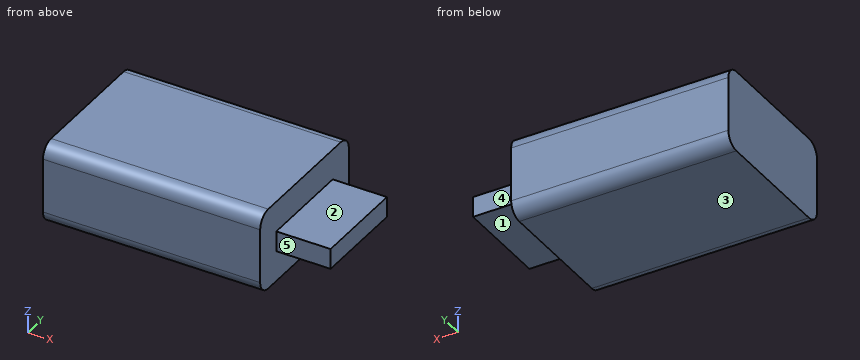
```python
from build123d import *

# Parameters (mm, degrees)
SKICA1_W                = 16
SKICA1_H                = 11
P_IDAT_VYSUNUT_M1_DEPTH = 6
ZAOBLIT1_R              = 1
SKICA2_W                = 1.5
SKICA2_H                = 7
P_IDAT_VYSUNUT_M2_DEPTH = 4


with BuildPart() as part:
    # Skica1 → Přidat vysunutím1 (new body)
    with BuildSketch(Plane.XY):
        Rectangle(SKICA1_W, SKICA1_H)
    extrude(amount=P_IDAT_VYSUNUT_M1_DEPTH)

    # Zaoblit1
    zaoblit1_edges = [part.edges().sort_by_distance(p)[0] for p in [
        (0, -5.5, 6),
        (0, -5.5, 0),
        (0, 5.5, 0),
        (0, 5.5, 6),
    ]]
    fillet(zaoblit1_edges, radius=ZAOBLIT1_R)

    # Skica2 → Přidat vysunutím2 (add)
    with BuildSketch(Plane(origin=(8, 0, 0), x_dir=(0, 0, -1), z_dir=(1, 0, 0))):
        with Locations((-3, 0)):
            Rectangle(SKICA2_W, SKICA2_H)
    extrude(amount=P_IDAT_VYSUNUT_M2_DEPTH)


solid = part.part
```
CAD build for the part. Positions are in the model's coordinates, mm. Face numbers are marked on the shaded views. A direction names the side the tool comes from. Round coordinates to 2 decimals unless told otherwise and drop trailing zeros. Write each loop counter-clockwise with the first axis right and the second up, starting at its lowest first coordinate (ties: lowest second). Pieces come first, ordered by that corner, then holes. Notation, with made-up numbers: (43, -31.5) - (72, -31.5) arc R27 cw to (72, -12.5) - close; hole circle Ø11 at (37, -24). An arc over 180 degrees is marked (long way). Return JSON: item names as keys, results as strings. Group by question number.
Item 1: Band-saw the part on C-C on y = 3.75. List the corners of the cut face in (x, z).
Item 2: Flat gauge pins, fed straight in: pin 1 Ø3 at (x, y) = (11, 0) entering from +Z; pin 2 Ø0.8 at (x, z) = (10.5, 3) entering from +Y; pin 3 Ø3 at (y, z) = (1.5, 1.5) entering from +X; pin 4 Ø2 at (x, y) = (11, -1.5) entering from -Z. Where does each tip first touch, or does it go through?
Item 3: Probe probe 1 along X at (y, z) = (3.5, 2); probe 2 along Z at (x, y) = (10.25, -3); probe 3 along Y at (x, z) = (-2.5, 5.15). List the from-to ranges inside material, lowest first.
Item 4: Band-saw the part on D-D on z = 1.3. List the corners of the cut face in (x, y).
Item 5: Band-saw the part on B-B on z = 2.55. List the corners of the cut face in (x, y), plus the area to 3 significant figures.
Item 6: 3-axis set-ups, long thin cutter, end or side, ignore diameter. For the marked faces 1, 2, 3, 4 and 5: which of +Z, -Z, +X, -X, +Y, -Y reach the whole face in a straight line?
Item 7: Band-saw the part on A-A on y = -1.25. List the corners of the cut face in (x, z), plus the area to 3 significant figures.
Resolved:
{
 "1": {"outline": "(-8, 0) - (8, 0) - (8, 6) - (-8, 6) - close"},
 "2": {"pin 1": "stops at z = 3.75", "pin 2": "stops at y = 3.5", "pin 3": "stops at x = 12", "pin 4": "stops at z = 2.25"},
 "3": {"probe 1": "x = -8 to 8", "probe 2": "z = 2.25 to 3.75", "probe 3": "y = -5.49 to 5.49"},
 "4": {"outline": "(-8, -5.5) - (8, -5.5) - (8, 5.5) - (-8, 5.5) - close"},
 "5": {"outline": "(-8, -5.5) - (8, -5.5) - (8, -3.5) - (12, -3.5) - (12, 3.5) - (8, 3.5) - (8, 5.5) - (-8, 5.5) - close", "area": "204 mm²"},
 "6": {"face 1": "-Z, +X, +Y, -Y", "face 2": "+Z, +X, +Y, -Y", "face 3": "-Z, +X, -X, +Y, -Y", "face 4": "+Z, -Z, +X, +Y", "face 5": "+Z, -Z, +X, -Y"},
 "7": {"outline": "(-8, 0) - (8, 0) - (8, 2.25) - (12, 2.25) - (12, 3.75) - (8, 3.75) - (8, 6) - (-8, 6) - close", "area": "102 mm²"}
}
